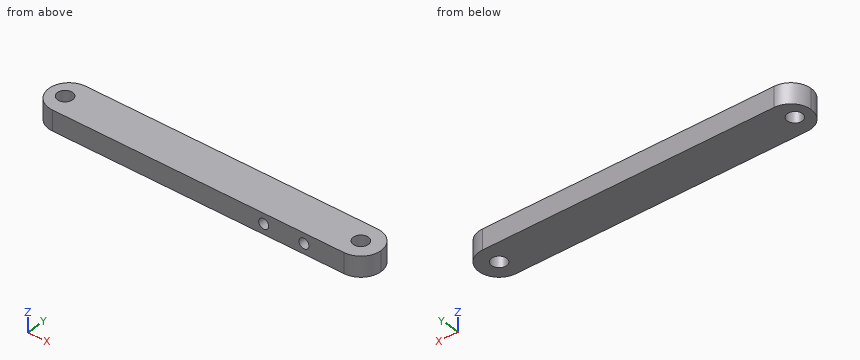
from build123d import *

# Parameters (mm, degrees)
SKETCH1_W           = 209.55
SKETCH1_H           = 12.7
BOSS_EXTRUDE1_DEPTH = 12.7
SKETCH2_R           = 4.7625
CUT_EXTRUDE1_DEPTH  = 107.303248422
FILLET1_R           = 12.7
SKETCH4_R           = 3.175
CUT_EXTRUDE3_DEPTH  = 12.7


with BuildPart() as part:
    # Sketch1 → Boss-Extrude1 (new, symmetric)
    with BuildSketch(Plane(origin=(0, 0, 0), x_dir=(1, 0, 0), z_dir=(0, 1, 0))):
        Rectangle(SKETCH1_W, SKETCH1_H)
    extrude(amount=BOSS_EXTRUDE1_DEPTH, both=True)

    # Sketch2 → Cut-Extrude1 (cut, through all)
    with BuildSketch(Plane.XY.offset(6.35)):
        with Locations((-94.615, 0)):
            Circle(SKETCH2_R)
        with Locations((92.075, 0)):
            Circle(SKETCH2_R)
    extrude(amount=-CUT_EXTRUDE1_DEPTH, mode=Mode.SUBTRACT)

    # Fillet1
    fillet1_edges = [part.edges().sort_by_distance(p)[0] for p in [
        (104.775, -12.7, 0),
        (104.775, 12.7, 0),
        (-104.775, -12.7, 0),
        (-104.775, 12.7, 0),
    ]]
    fillet(fillet1_edges, radius=FILLET1_R - 0.0001)  # a hair under: the kernel refuses the full size

    # Sketch4 → Cut-Extrude3 (cut)
    with BuildSketch(Plane.XZ.offset(12.7)):
        with Locations(Location((41.275, 0, 0), (0, 0, 270))):
            Circle(SKETCH4_R)
        with Locations(Location((66.675, 0, 0), (0, 0, 270))):
            Circle(SKETCH4_R)
    extrude(amount=-CUT_EXTRUDE3_DEPTH, mode=Mode.SUBTRACT)


solid = part.part
Input: part model. Units: mm. Frame: model coordinates. Give positions to 0.01 mm unless a question says otherwise; leave off trailing zeros. Write each loop counter-clockwise with the first axis right and the second up, starting at its lowest first coordinate (ties: lowest second). Pieces come first, ordered by that corner, then holes. Notation, with made-up numbers: M 65,24 L 117,24 A15 ccw 117,49 Z; hole C -15.75,-31 d1. An arc over 180 degrees is marked long. Write item = value, one per line. Start each with the question number.
1) Cut plane B-B on y = 3. Return the cut outline in (x, z).
2) Cut plane A-A on z = 0. Count the separate pieces of the cut face and the enclosed holes in it, then the cut area to 3 significant figures.
3) First-contact query: pin 1 Ø11 at (x, y) = (92.075, 0) entering from -Z; pin 2 Ø8.5 at (x, y) = (-94.615, 0) entering from -Z; pin 3 Ø5 at (y, z) = (8.5, 2.5) entering from -X; pin 4 Ø4 at (x, z) = (66.675, 0) entering from -Y. Flat tips, straight axial feed; report the tip coordinate or a pass-through.
4) Material intervals for line 1 along X through (y, z) = (-0.5, 4.75); line 2 along X through (y, z) = (-7.5, 0); line 3 along X through (y, z) = (-4.25, 0), sorted ascending. Write a range as [from, to].
Solved:
q1.outline = M -104.42,-6.35 L -98.31,-6.35 L -98.31,6.35 L -104.42,6.35 Z; M -90.92,-6.35 L 88.38,-6.35 L 88.38,6.35 L -90.92,6.35 Z; M 95.77,-6.35 L 104.42,-6.35 L 104.42,6.35 L 95.77,6.35 Z
q2.separate_pieces = 1
q2.enclosed_holes = 2
q2.area = 4,880 mm2
q3.pin_1 = -6.35
q3.pin_2 = through
q3.pin_3 = -103.27
q3.pin_4 = 0
q4.line_1 = [-104.77, -99.35], [-89.88, 87.34], [96.81, 104.77]
q4.line_2 = [-102.32, 38.1], [44.45, 63.5], [69.85, 102.32]
q4.line_3 = [-104.04, -96.76], [-92.47, 38.1], [44.45, 63.5], [69.85, 89.93], [94.22, 104.04]
